from build123d import *

# Parameters (mm, degrees)
BASEHEAD_DEPTH = 13
BEARINGSKE_W   = 0.8
BEARINGSKE_H   = 2.320508076


with BuildPart() as part:
    # HeadSke → BaseHead (new body)
    with BuildSketch(Plane(origin=(0, 0, 0), x_dir=(0, 0, -1), z_dir=(1, 0, 0))):
        Polygon((15, 8.660254038), (15, -8.660254038), (0, -17.320508076), (-15, -8.660254038), (-15, 8.660254038), (0, 17.320508076), align=None)
    extrude(amount=BASEHEAD_DEPTH)

    # BodySke → BaseBody (revolve)
    with BuildSketch(Plane.XY, mode=Mode.PRIVATE) as basebody_sk:
        Polygon((0, 0), (163, 0), (163, 8.626), (161.626, 10), (0, 10), align=None)
    revolve(basebody_sk.sketch.rotate(Axis((0, 0, 0), (1, 0, 0)), 90), axis=Axis((0, 0, 0), (1, 0, 0)))

    # Sketch3 → HeadChamfer (revolve, cut)
    with BuildSketch(Plane(origin=(0, 0, 0), x_dir=(1, 0, 0), z_dir=(0, 1, 0))):
        Polygon((3.75, 21.495190528), (-3.75, 8.504809472), (-15.804766255, 15.464632014), (-8.304766255, 28.455013071), align=None)
    revolve(axis=Axis((0, 0, 0), (1, 0, 0)), mode=Mode.SUBTRACT)

    # BearingSke → BearingFace (revolve, cut)
    with BuildSketch(Plane.XY, mode=Mode.PRIVATE) as bearingface_sk:
        with Locations((12.6, 16.160254038)):
            Rectangle(BEARINGSKE_W, BEARINGSKE_H)
    revolve(bearingface_sk.sketch.rotate(Axis((0, 0, 0), (1, 0, 0)), 270), axis=Axis((0, 0, 0), (1, 0, 0)), mode=Mode.SUBTRACT)


solid = part.part
Work out the finished part from the listing and answer in its coordinate system (mm). A direction names the side the tool comes from. Round coordinates to 2 decimals unless told otherwise and drop trailing zeros. Order: outer loops, then holes, each group sorted by start corner. A loop starts at its lowest first (then second) coordinate and runs counter-clockwise, first axis right, second up. Notation, with made-up numbers: M -20.5,76.25 L -15.5,76.25 A12 ccw -15.5,88.25 Z; hole C 49.5,5.25 d10. An arc over 180 degrees is marked long. Put each result on its own line as item: value. Start each with the question number.
Q1. Section A-A, the plane x = 17 is taken. Write down the section's boundary in (y, z).
Q2. Straight lines are drawn through the part: L1, parallel to Y at x = 116.5, z = 0; L2, parallel to X at y = -10, z = 5; L3, parallel to Z at x = 21.5, y = -5. For each, find the intervals that lie inside material, in ascending order. Write a range as [from, to].
Q3. A tool of negligible diameter and unlimited length cuts with its end or side. For faces 1 (the flat face through (12.2, -8, -13)), 2 (the flat face through (12.2, 7.5, -13.5)), 3 (the flat face through (12.2, -15.5, 0)), from which of +Z, -Z, +X, -X, +Y, -Y can it reach the whole face along a straight path? Write none if from no direction.
Q4. Flat-ended cylindrical pins translate along their axes: pin 1 (10 mm diameter, centred on y = -12.5, z = 5.5, fed in from +X); pin 2 (8 mm diameter, centred on y = 7, z = -12.5, fed in from +X); pin 3 (4 mm diameter, centred on x = 33.5, y = -1, fed in from +Z). Find the tip coordinate at first contact, or state that the pin passes through.
Findings below:
1. outline: C 0,0 d20
2. L1: y = [-10, 10]
2. L2: x = [0, 13]
2. L3: z = [-8.66, 8.66]
3. face 1: -Z, +X, -Y
3. face 2: -Z, +X, +Y
3. face 3: +X, -Y
4. pin 1: stops at x = 162.97
4. pin 2: stops at x = 13
4. pin 3: stops at z = 10
